Geometry: see drawing. Coordinates: mm, zero at the bounding-box minimum. A direction names the side the tool comes from. Coordinates: 2 decimals unless noted, no trailing zeros. Loops run counter-clockwise (first coordinate to the right, second up) from the corner with the lowest first, then second, coordinate; pieces in that order, holes last. Notation, with made-up numbers: (-8, 56.5) - (3, 56.5) arc R23 cw to (3, 94.5) - close; hole circle Ø5 at (50, 71.25). An arc over 180 degrees is marked (long way). Answer in a Markdown table with one row per item.
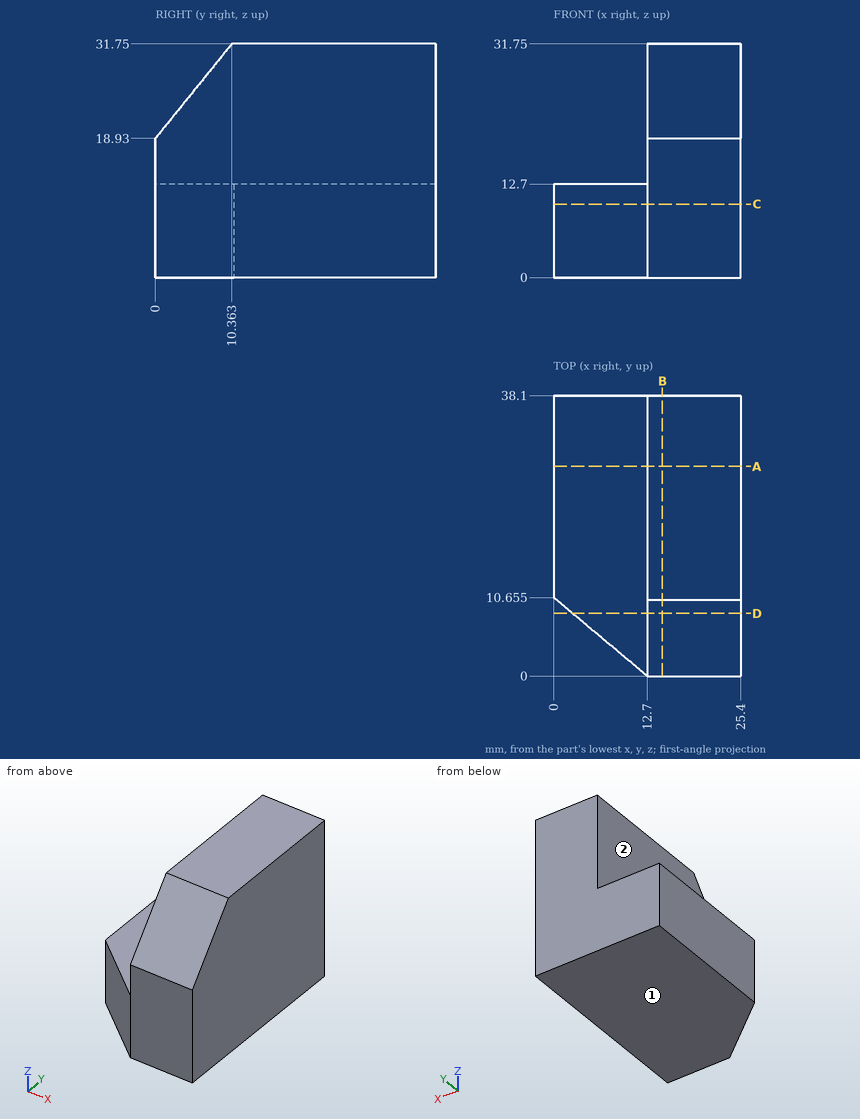
(1) Cut plane C-C on z = 10. Output: boundary loops of the cut face in (x, y) (1 decimal).
Verdict:
| item | result |
|---|---|
| outline | (0, 10.7) - (12.7, 0) - (25.4, 0) - (25.4, 38.1) - (0, 38.1) - close |
(2) First-contact query: pin 1 Ø14 at (x, y) = (4.5, 28.5) entering from +Z; pin 2 Ø1 at (y, z) = (31, 22) entering from -X. Flat tips, straight axial feed; report the tip coordinate or a pass-through.
Verdict:
| item | result |
|---|---|
| pin 1 | stops at z = 12.7 |
| pin 2 | stops at x = 12.7 |
(3) Access query for the marked faces 1 and 2. Directions: +Z, -Z, +X, -X, +Y, -Y. A direction counts if a zero-diameter tool reaches every point of the face in a straight line with its end or side. Return the directions, or none.
Verdict:
| item | result |
|---|---|
| face 1 | -Z, +X, -X, +Y, -Y |
| face 2 | +Z, -X, +Y, -Y |
(4) Cut plane B-B on x = 14.75. Output: boundary loops of the cut face in (y, z).
Verdict:
| item | result |
|---|---|
| outline | (0, 0) - (38.1, 0) - (38.1, 31.75) - (10.36, 31.75) - (0, 18.93) - close |
(5) Cut plane D-D on y = 8.5. Output: boundary loops of the cut face in (x, z) (1 decimal).
Verdict:
| item | result |
|---|---|
| outline | (2.6, 0) - (25.4, 0) - (25.4, 29.4) - (12.7, 29.4) - (12.7, 12.7) - (2.6, 12.7) - close |
(6) Ray query, probe 1 along Z at (x, y) = (11.75, 20.5); probe 2 along X at (y, z) = (14, 26.5); probe 3 along Y at (x, z) = (14.25, 24). Return the intervals inside material, ascending.
Verdict:
| item | result |
|---|---|
| probe 1 | z = 0 to 12.7 |
| probe 2 | x = 12.7 to 25.4 |
| probe 3 | y = 4.1 to 38.1 |
(7) Cut plane A-A on y = 28.5. Output: boundary loops of the cut face in (x, z).
Verdict:
| item | result |
|---|---|
| outline | (0, 0) - (25.4, 0) - (25.4, 31.75) - (12.7, 31.75) - (12.7, 12.7) - (0, 12.7) - close |
